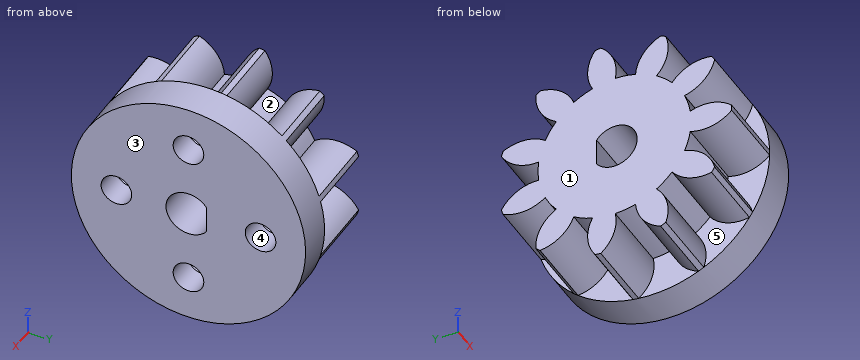
from build123d import *

# Parameters (mm, degrees)
BASPROSKE_W                  = 8
BASPROSKE_H                  = 13
TOOTHCUT_DEPTH               = 21.049937656
TEETHCUTS_COUNT              = 11
TEETHCUTS_ANGLE              = 327.272727273
BORSKE_R                     = 0.4
BORE_DEPTH                   = 50.0000508
ESTRUSIONE_ESTRUSIONE1_START = 4
SCHIZZO2_R                   = 13
ESTRUSIONE_ESTRUSIONE1_DEPTH = 4
TAGLIO_ESTRUSIONE1_DEPTH     = 14
FORO_PER_VITE_M3_1_D         = 3.4
FORO_PER_VITE_M3_1_DEPTH     = 3
FORO_PER_VITE_M3_1_TIP       = 1.021463052


with BuildPart() as part:
    # BasProSke → Base-Revolve (revolve)
    with BuildSketch(Plane(origin=(0, 0, 0), x_dir=(1, 0, 0), z_dir=(0, 1, 0)), mode=Mode.PRIVATE) as base_revolve_sk:
        with Locations((4, 6.5)):
            Rectangle(BASPROSKE_W, BASPROSKE_H)
    revolve(base_revolve_sk.sketch.rotate(Axis((-10, 0, 0), (1, 0, 0)), 180), axis=Axis((-10, 0, 0), (1, 0, 0)))

    # TooCutSke → ToothCut (cut, through all)
    with BuildSketch(Plane(origin=(0, 0, 0), x_dir=(0, 0, -1), z_dir=(1, 0, 0))):
        with BuildLine():
            ThreePointArc((1.139858048, 8.422216135), (0, 8.499), (-1.139858048, 8.422216135))
            ThreePointArc((-1.139858048, 8.422216135), (-1.658602184, 10.826907356), (-3.387115532, 12.577300725))
            ThreePointArc((-3.387115532, 12.577300725), (0, 13.0254), (3.387115532, 12.577300725))
            ThreePointArc((3.387115532, 12.577300725), (1.658602184, 10.826907356), (1.139858048, 8.422216135))
        make_face()
    toothcut = extrude(amount=TOOTHCUT_DEPTH, mode=Mode.SUBTRACT)

    # TeethCuts: ToothCut ×11 about axis
    teethcuts_axis = Axis((-10, 0, 0), (1, 0, 0))
    for i in range(1, TEETHCUTS_COUNT):
        add(toothcut.rotate(teethcuts_axis, i * TEETHCUTS_ANGLE / (TEETHCUTS_COUNT - 1)), mode=Mode.SUBTRACT)

    # BorSke → Bore (cut, symmetric)
    with BuildSketch(Plane(origin=(0, 0, 0), x_dir=(0, 0, -1), z_dir=(1, 0, 0))):
        with Locations(Location((0, 0, 0), (0, 0, 180))):
            Circle(BORSKE_R)
    extrude(amount=BORE_DEPTH, both=True, mode=Mode.SUBTRACT)

    # Schizzo2 → Estrusione-Estrusione1 (add)
    with BuildSketch(Plane(origin=(8, 0, 0), x_dir=(0, 0, -1), z_dir=(1, 0, 0)).offset(ESTRUSIONE_ESTRUSIONE1_START)):
        with Locations(Location((0, 0, 0), (0, 0, 173.223714884))):
            Circle(SCHIZZO2_R)
    extrude(amount=-ESTRUSIONE_ESTRUSIONE1_DEPTH)

    # Schizzo1 → Taglio-Estrusione1 (cut)
    with BuildSketch(Plane(origin=(12, 0, 0), x_dir=(0, 0, -1), z_dir=(1, 0, 0))):
        with BuildLine():
            Line((-1.5, 2), (1.5, 2))
            ThreePointArc((1.5, 2), (0, -2.5), (-1.5, 2))
        make_face()
    extrude(amount=-TAGLIO_ESTRUSIONE1_DEPTH, mode=Mode.SUBTRACT)

    # Foro per Vite M3-1
    with Locations(Plane(origin=(12, 0, 0), x_dir=(0, 0, -1), z_dir=(1, 0, 0))):
        with Locations((0, 8), (8, 0), (0, -8), (-8, 0)):
            Hole(FORO_PER_VITE_M3_1_D / 2, depth=FORO_PER_VITE_M3_1_DEPTH)
            with Locations((0, 0, -(FORO_PER_VITE_M3_1_DEPTH + FORO_PER_VITE_M3_1_TIP / 2))):  # 118° drill point
                Cone(0, FORO_PER_VITE_M3_1_D / 2, FORO_PER_VITE_M3_1_TIP, mode=Mode.SUBTRACT)


solid = part.part
Check sheet for the modelled part. Datum: model origin and axes. Units: mm. Face numbers are marked on the shaded views. A direction names the side the tool comes from. Give positions to 0.01 mm unless a question says otherwise; leave off trailing zeros. Order: outer loops, then holes, each group sorted by start corner. A loop starts at its lowest first (then second) coordinate and runs counter-clockwise, first axis right, second up. Notation, with made-up numbers: M 78,8 L 136,8 A7 cw 136,16 Z; hole C -1.5,-6.75 d9. An arc over 180 degrees is marked long. Answer as CSV lines item,"result". Start each with the question number.
Item 1: Cross-section at C-C on z = -10.5. Enter the section's corners in (x, y).
Item 2: Tool access check on the marked faces 3, 4 and 5. Record the directions out of +Z, -Z, +X, -X, +Y, -Y that give a thin tool (end or side, any length) a straight path to the whole face; none if there is none.
Item 3: Gauge pin test, flat ends, axial feed: P1, Ø5.5, axis at y = -0.5, z = -10.5, coming from the -X side; P2, Ø4, axis at x = 4, z = 2, coming from the +Y side; P3, Ø1.8, axis at y = -7.5, z = -8.5, coming from the -X side; P4, Ø2, axis at y = 0, z = 8, coming from the +X side. Record the tip position at first contact, or that the pin passes through.
Item 4: Thickness scan on line 1 (Y direction, x = 9.95, z = 0); line 2 (Z direction, x = 10.2, y = 0); line 3 (Y direction, x = 1, z = -9.25). Record the ranges inside material, lowest first. Write a range as [from, to].
Item 5: Cross-section at B-B on z = 3. Enter the section's corners in (x, y), plus the area to 3 significant figures.
Item 6: Cross-section at A-A on y = -4. Enter the section's corners in (x, z), plus the area to 3 significant figures.
Item 7: Mould release check, pull along Z, two halves, no side actions. Record for the marked faces 1 and 2: +Z half, -Z half, draft (parallel to the pull), parting line (faces both ways), or undercut.
Established:
1,outline,"M 0,-5.93 L 8,-5.93 L 8,-7.66 L 12,-7.66 L 12,7.66 L 8,7.66 L 8,2.99 L 0,2.99 L 0,-0.04 L 8,-0.04 L 8,-3.2 L 0,-3.2 Z"
2,face 3,"+Z, -Z, +X, +Y, -Y"
2,face 4,"+X"
2,face 5,"-X"
3,P1,"stops at x = 0"
3,P2,"stops at y = 12.56"
3,P3,"stops at x = 8"
3,P4,"stops at x = 8.58"
4,line 1,"y = [-13, -9.7], [-6.3, -2.5], [2, 6.3], [9.7, 13]"
4,line 2,"z = [-13, -9.7], [-6.3, -2.5], [2.5, 6.3], [9.7, 13]"
4,line 3,"y = [-5.83, -2.54], [-0.17, 2.89], [6.13, 8.76]"
5,outline,"M 0,-7.95 L 8,-7.95 L 8,-12.65 L 12,-12.65 L 12,12.65 L 8,12.65 L 8,12.33 L 0,12.33 Z"
5,area,"263 mm^2"
6,outline,"M 0,-11.32 L 8,-11.32 L 8,-12.37 L 12,-12.37 L 12,12.37 L 8,12.37 L 8,11.32 L 0,11.32 Z"
6,area,"280 mm^2"
7,face 1,"draft"
7,face 2,"undercut"
